from build123d import *

# Parameters (mm, degrees)
F0_W     = 70
F0_H     = 12
F1_DEPTH = 50
F2_DEPTH = 12


with BuildPart() as f1:
    # F0 (on Front) → F1 (new body)
    with BuildSketch(Plane.XZ):
        with Locations((-0.595462, -17.008216)):
            Rectangle(F0_W, F0_H)
    extrude(amount=F1_DEPTH)

    # F0 (on Front) → F2 (join)
    with BuildSketch(Plane.XZ):
        with BuildLine():
            ThreePointArc((6, 16.991784), (4.242641, 21.234424), (0, 22.991784))
            ThreePointArc((0, 22.991784), (-4.242641, 12.749143), (6, 16.991784))
        make_face()
        Polygon((0, 36.991784), (-35.595462, 36.991784), (-35.595462, -11.008216), (34.404538, -11.008216), (34.404538, 36.991784), align=None)
        with BuildLine():
            ThreePointArc((6, 16.991784), (-4.242641, 12.749143), (0, 22.991784))
            ThreePointArc((0, 22.991784), (4.242641, 21.234424), (6, 16.991784))
        make_face(mode=Mode.SUBTRACT)
        with Locations((-0.595462, -17.008216)):
            Rectangle(F0_W, F0_H)
    extrude(amount=F2_DEPTH)


solid = f1.part
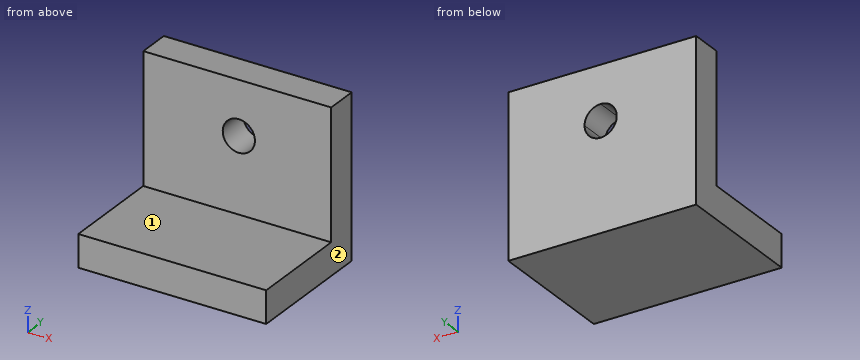
Part model, mm, in its own coordinate system. Face numbers are marked on the shaded views. A direction names the side the tool comes from. Round coordinates to 2 decimals unless told otherwise and drop trailing zeros. Write each loop counter-clockwise with the first axis right and the second up, starting at its lowest first coordinate (ties: lowest second). Pieces come first, ordered by that corner, then holes. Notation, with made-up numbers: M -27,60 L 18,60 A22 ccw 18,88 Z; hole C 2,-26.5 d5. An arc over 180 degrees is marked long. Return JSON: item names as keys, results as strings. Group by question number.
(1) Saw through at C-C on y = -27.5. Write the cut outline in (x, z), then the cut area to 3 significant figures.
(2) Saw through at A-A on z = 13.5. Write the cut outline in (x, y).
(3) Drill centre lines: probe 1 along Y at (x, z) = (-10, 3); probe 2 along Z at (x, y) = (31.5, -28.5); probe 3 along X at (y, z) = (-4.5, 14). Where is each one in solid material? Low to high.
(4) Which spindle directions (+Z, -Z, +X, -X, +Y, -Y) get a long thin tool onto all of the face, cutting with end or side? Do the marked faces 1 and 2. Say none if no direction does.
(5) Pin check, flat tips, straight feed: pin 1 Ø4 at (x, z) = (-4, 0) entering from -Y; pin 2 Ø4 at (x, y) = (-8, -18) entering from +Z. Stop position of each tip, or through.
(6) Saw through at B-B on x = -31. Write the cut outline in (y, z).
Returned:
{
 "1": {"outline": "M -35.6,-23.01 L 34.4,-23.01 L 34.4,-11.01 L -35.6,-11.01 Z", "area": "840 mm²"},
 "2": {"outline": "M -35.6,-12 L -4.88,-12 L -4.88,0 L -35.6,0 Z; M 4.88,-12 L 34.4,-12 L 34.4,0 L 4.88,0 Z"},
 "3": {"probe 1": "-12 to 0", "probe 2": "-23.01 to -11.01", "probe 3": "-35.6 to -5.2, 5.2 to 34.4"},
 "4": {"face 1": "+Z, +X, -X, -Y", "face 2": "+Z, -Z, +X, +Y, -Y"},
 "5": {"pin 1": "y = -12", "pin 2": "z = -11.01"},
 "6": {"outline": "M -50,-23.01 L 0,-23.01 L 0,36.99 L -12,36.99 L -12,-11.01 L -50,-11.01 Z"}
}
